Input: part model. Units: mm. Frame: model coordinates. Face numbers are marked on the shaded views. A direction names the side the tool comes from. Coordinates: 2 decimals unless noted, no trailing zeros. Write each loop counter-clockwise with the first axis right and the second up, starting at its lowest first coordinate (ties: lowest second). Pieces come first, ordered by that corner, then holes. Notation, with made-up numbers: (6.25, -17) -> (24.25, -17) arc R31 cw to (24.25, 11) -> close; hole circle Ø7 at (37, 29.25). An arc over 180 degrees is marked (long way). One line per question, with ' | ' between items. Start each with the question number.
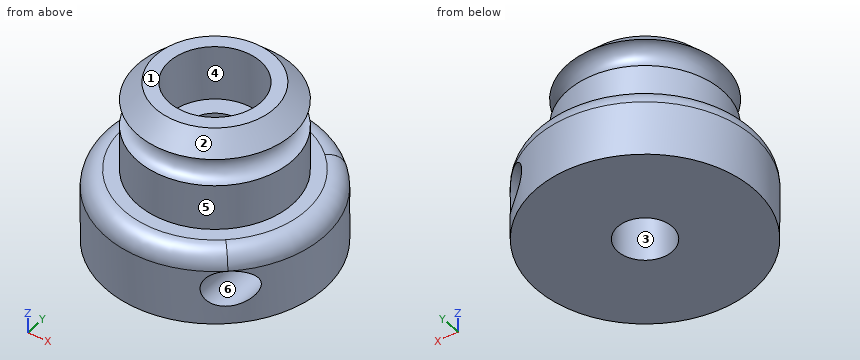
```python
from build123d import *

# Parameters (mm, degrees)
F2_SIZE        = 1.99999
F3_R           = 5
F4_DEPTH       = 6
F5_R           = 12
F6_DEPTH       = 8
F7_R           = 3
F8_DEPTH       = 12
F9_R           = 2
F10_DEPTH      = 12.001
F10_DEPTH_BACK = 12.001
F11_R          = 2


# Not quite as in the source:
# - a fillet or chamfer is up to 0.001 mm smaller than in the source, because OpenCascade refuses the exact size


with BuildPart() as f1:
    # F0 (on Right) → F1 (revolve)
    with BuildSketch(Plane.YZ):
        with BuildLine():
            Line((-8.5, 0), (0, 0))
            Line((0, 0), (0, 10))
            Line((0, 10), (-8.5, 10))
            Line((-8.5, 10), (-8.5, 8))
            ThreePointArc((-8.5, 8), (-7, 6.5), (-8.5, 5))
            Line((-8.5, 5), (-8.5, 0))
        make_face()
    revolve(axis=Axis((0, 0, 5), (0, 0, -1)))

    # F2 (size 2 in the source; OpenCascade refuses exactly that, so slightly less here)
    f2_edges = [f1.edges().sort_by_distance(p)[0] for p in [
        (0, 8.5, 10),
    ]]
    chamfer(f2_edges, length=F2_SIZE)

    # F3 (on face) → F4 (cut)
    with BuildSketch(Plane.XY.offset(10)):
        Circle(F3_R)
    extrude(amount=-F4_DEPTH, mode=Mode.SUBTRACT)

    # F5 (on face) → F6 (join)
    with BuildSketch(Plane(origin=(0, 0, 0), x_dir=(1, 0, 0), z_dir=(0, 0, -1))):
        Circle(F5_R)
    extrude(amount=F6_DEPTH)

    # F7 (on face) → F8 (cut, through all)
    with BuildSketch(Plane.XY.offset(4)):
        Circle(F7_R)
    extrude(amount=-F8_DEPTH, mode=Mode.SUBTRACT)

    # F9 (on Front) → F10 (cut, two sides)
    with BuildSketch(Plane.XZ) as f10_sk:
        with Locations((8, -4)):
            Circle(F9_R)
    extrude(amount=-F10_DEPTH, mode=Mode.SUBTRACT)
    extrude(f10_sk.sketch, amount=F10_DEPTH_BACK, mode=Mode.SUBTRACT)

    # F11
    f11_edges = [f1.edges().sort_by_distance(p)[0] for p in [
        (-12, 0, 0),
    ]]
    fillet(f11_edges, radius=F11_R)


solid = f1.part
```
1) Ray query, line 1 (Y direction, x = 0, z = -2.25); line 2 (Y direction, x = 0, z = 0.5); line 3 (X direction, y = -1, z = -3.25). Return the intervals inside material, ascending.
2) First-contact query: P1, Ø6, axis at y = 8.5, z = -1.5, coming from the -X side; P2, Ø8, axis at y = 4.5, z = 6, coming from the -X side; P3, Ø1.5, axis at x = -6.5, z = 2.5, coming from the +Y side; P4, Ø2.5, axis at x = 8, z = -4, coming from the +Y side. Flat tips, straight axial feed; report the tip coordinate or a pass-through.
3) Pull-direction query (X, two-part tool) for the marked faces 1, 2, 3 and 4; classes: released by +X, released by -X, zero draft, split by the parting line, or undercut.
4) Access query for the marked faces 5 and 6. Directions: +Z, -Z, +X, -X, +Y, -Y. A direction counts if a zero-diameter tool reaches every point of the face in a straight line with its end or side. Return the directions, or none.
5) Section C-C, the plane z = -4. Return loops of the section in (x, y).
6) Section A-A, the plane y = 0. Give the number of separate pieces and of enclosed holes in the cut face, then the cut area to 3 significant figures.
7) Section D-D, the plane z = 3.5. Return loops of the section in (x, y).
Answer block:
1) line 1: y = -12 to -3, 3 to 12 | line 2: y = -8.5 to -3, 3 to 8.5 | line 3: x = -11.96 to -2.83, 2.83 to 6.15, 9.85 to 11.96
2) P1: stops at x = -10.65 | P2: stops at x = -8.48 | P3: stops at y = 6.26 | P4: passes through
3) face 1: zero draft | face 2: split by the parting line | face 3: undercut | face 4: undercut
4) face 5: +Z | face 6: +Y, -Y
5) outline: (6, -10.39) -> (6, 10.39) arc R12 ccw (long way) to start; (10, -6.63) arc R12 ccw to (10, 6.63) -> close; hole circle Ø6 at (0, 0)
6) separate pieces: 2 | enclosed holes: 1 | area: 205 mm2
7) outline: circle Ø17 at (0, 0); hole circle Ø6 at (0, 0)
